```python
from build123d import *

# Parameters (mm, degrees)
CHAMFER1_SIZE      = 1.5
FILLET1_R          = 1.5
SKETCH3_W          = 23.767877036
SKETCH3_H          = 3
CUT_EXTRUDE1_DEPTH = 1.5


with BuildPart() as part:
    # Sketch1 → Revolve1 (revolve)
    with BuildSketch(Plane.XY):
        Polygon((0, 0), (0, 11), (5, 11), (5, 8), (25, 8), (25, 6), (38, 6), (38, 0), align=None)
    revolve(axis=Axis((-97.318857056, 0, 0), (1, 0, 0)))

    # Chamfer1
    chamfer1_edges = [part.edges().sort_by_distance(p)[0] for p in [
        (38, -6, 0),
    ]]
    chamfer(chamfer1_edges, length=CHAMFER1_SIZE)

    # Fillet1
    fillet1_edges = [part.edges().sort_by_distance(p)[0] for p in [
        (0, -11, 0),
    ]]
    fillet(fillet1_edges, radius=FILLET1_R)

    # Sketch3 → Cut-Extrude1 (cut)
    with BuildSketch(Plane.ZY):
        Rectangle(SKETCH3_W, SKETCH3_H)
    extrude(amount=-CUT_EXTRUDE1_DEPTH, mode=Mode.SUBTRACT)


solid = part.part
```
For this review, take the finished solid that the model builds, in its own axes (mm). A direction names the side the tool comes from. Round coordinates to 2 decimals unless told otherwise and drop trailing zeros. Write each loop counter-clockwise with the first axis right and the second up, starting at its lowest first coordinate (ties: lowest second). Pieces come first, ordered by that corner, then holes. Notation, with made-up numbers: (74.25, 34) -> (103.25, 34) arc R15 cw to (103.25, 45) -> close; hole circle Ø6 at (84, 73). An arc over 180 degrees is marked (long way). One line per question, with ' | ' between items. Start each with the question number.
1) Wall thickness on line 1 along X through (y, z) = (4.5, -7.5); line 2 along Y through (x, z) = (22, -0.25); line 3 along X through (y, z) = (-6.5, -0.25): over which ranges is each line inside the solid? List them lowest first.
2) Add section B-B (y = 0). Write out the cut boundary in (x, z), and give its area (3 significant figures).
3) For pin 1 Ø4 at (x, z) = (17, -3.5) entering from +Y; pin 2 Ø0.8 at (x, z) = (0.5, -5) entering from +Y; pin 3 Ø8 at (x, z) = (22, 1) entering from -Y, all flat-tipped, find the tip position at first contact; note any pin that passes through.
4) Add section D-D (x = 4). Write out the cut boundary in (y, z), and give its area (3 significant figures).
5) Machinability: for faces 5 (the flat face through (5, -2, -8)), 6 (the flat face through (0, -5, 0)), 7 (the flat face through (1, 1.5, 0)), which of the approach directions +Z, -Z, +X, -X, +Y, -Y give a long, thin tool a straight path to every point of the face, cutting with its end or side? Answer none if there is none.
6) Mouldability with a two-part tool opening along Y and no side actions: class faces 1 (the flat face through (1.5, 0, 0)), 2 (the flat face through (1, -1.5, 0)), 3 (the flat face through (38, 0, 0)), 4 (the cylindrical face through (3.27, -2.38, -10.74)) as +Y half, -Y half, draft (parallel to the pull), parting line (faces both ways), or undercut.
7) Add section A-A (z = 0). Write out the cut boundary in (x, y).
8) Add section C-C (x = 15.5). Write out the cut boundary in (y, z), and give its area (3 significant figures).
Reported:
1) line 1: x = 0 to 5 | line 2: y = -8 to 8 | line 3: x = 0 to 25
2) outline: (1.5, -11) -> (5, -11) -> (5, -8) -> (25, -8) -> (25, -6) -> (36.5, -6) -> (38, -4.5) -> (38, 4.5) -> (36.5, 6) -> (25, 6) -> (25, 8) -> (5, 8) -> (5, 11) -> (1.5, 11) -> close | area: 551 mm²
3) pin 1: stops at y = 7.86 | pin 2: stops at y = 9.74 | pin 3: stops at y = -8
4) outline: circle Ø22 at (0, 0) | area: 380 mm²
5) face 5: +X | face 6: +Z, -Z, -X, +Y, -Y | face 7: +Z, -Z, -X
6) face 1: undercut | face 2: undercut | face 3: draft | face 4: parting line
7) outline: (0, -9.5) arc R1.5 ccw to (1.5, -11) -> (5, -11) -> (5, -8) -> (25, -8) -> (25, -6) -> (36.5, -6) -> (38, -4.5) -> (38, 4.5) -> (36.5, 6) -> (25, 6) -> (25, 8) -> (5, 8) -> (5, 11) -> (1.5, 11) arc R1.5 ccw to (0, 9.5) -> (0, 1.5) -> (1.5, 1.5) -> (1.5, -1.5) -> (0, -1.5) -> close
8) outline: circle Ø16 at (0, 0) | area: 201 mm²
